Autodesk Inventor part; units mm, degrees
ref_plane "YZ Plane" through (0, 0, 0) normal (1, 0, 0) x (0, 1, 0)
ref_plane "XZ Plane" through (0, 0, 0) normal (0, 1, 0) x (-1, 0, 0)
ref_plane "XY Plane" through (0, 0, 0) normal (0, 0, 1) x (1, 0, 0)
sketch "Sketch1" plane through (0, 0, 0) normal (0, 1, 0) x (-1, 0, 0)
  circle A0 centre (0, -139.7) radius 3.3782
  line L0 (6.35, -37.5671) -> (6.35, -393.6488)
  line L1 (-6.35, -37.5671) -> (-6.35, -393.7)
  circle A1 centre (193.0245, -202.0047) radius 3.3782
  circle A2 centre (202.0047, -193.0245) radius 3.3782
  line L2 (269.2628, -287.2233) -> (16.4197, -34.3803)
  line L3 (287.2233, -269.2628) -> (34.3803, -16.4197)
  circle A3 centre (94.1906, -103.1708) radius 3.3782
  circle A4 centre (103.1708, -94.1906) radius 3.3782
  circle A5 centre (139.7, 0) radius 3.3782
  line L4 (133.35, 0) -> (133.35, 6.35)
  line L5 (273.05, 6.35) -> (273.05, 0)
  line L6 (37.5671, -6.35) -> (393.6488, -6.35)
  line L7 (37.5671, 6.35) -> (393.7, 6.35)
  line L8 (146.05, 0) -> (146.05, 6.35)
  circle A6 centre (277.5195, -270.2276) radius 3.3782
  circle A7 centre (270.2276, -277.5195) radius 3.3782
  arc A8 (269.2628, -287.2233) -> (287.2233, -269.2628) centre (0, 0) ccw
  circle A9 centre (0, -387.35) radius 3.3782
  arc A10 (0, -393.7) -> (6.35, -393.6488) centre (0, 0) ccw
  line L9 (-6.35, -393.7) -> (0, -393.7)
  circle A11 centre (0, -279.4) radius 3.3782
  arc A12 (6.35, -37.5671) -> (16.4197, -34.3803) centre (0, 0) ccw
  arc A13 (34.3803, -16.4197) -> (37.5671, -6.35) centre (0, 0) ccw
  circle A14 centre (0, 0) radius 14.2875
  line L10 (38.1, 0) -> (38.1, 12.8556) construction
  arc A15 (-6.214, 37.5898) -> (-37.5898, 6.214) centre (0, 0) ccw
  arc A16 (37.5671, 6.35) -> (-6.35, -37.5671) centre (0, 0) ccw
  circle A17 centre (387.35, 0) radius 3.3782
  line L11 (393.7, 0) -> (393.7, 6.35)
  circle A18 centre (279.4, 0) radius 3.3782
  line L12 (285.75, 6.35) -> (285.75, 0)
  arc A19 (393.6488, -6.35) -> (393.7, 0) centre (0, 0) ccw
  line L13 (0, -285.75) -> (-6.35, -285.75)
  line L14 (-6.35, -273.05) -> (0, -273.05)
  circle A20 centre (0, -336.55) radius 3.3782
  circle A21 centre (241.5985, -234.3065) radius 3.3782
  circle A22 centre (234.3065, -241.5985) radius 3.3782
  circle A23 centre (336.55, 0) radius 3.3782
  dimension "d2" = 12.7
  dimension "d3" = 12.7
  dimension "d4" = 38.1
  dimension "d6" = 38.1
  dimension "d7" = 6.35
  dimension "d8" = 6.35
  dimension "d9" = 6.35
  dimension "d10" = 12.7
  dimension "d11" = 12.7
  dimension "d12" = 95.25
  dimension "d13" = 6.7564
  dimension "d14" = 6.7564
  dimension "d15" = 6.7564
  dimension "d16" = 6.35
  dimension "d17" = 6.7564
  dimension "d18" = 6.35
  dimension "d19" = 6.35
  dimension "d20" = 6.7564
  dimension "d21" = 6.7564
  dimension "d22" = 6.7564
  dimension "d23" = 6.35
  dimension "d24" = 6.7564
  dimension "d25" = 28.575
  dimension "d28" = 38.1
  dimension "d30" = 6.35
  dimension "d31" = 139.7
  dimension "d34" = 6.35
  dimension "d37" = 277.5195
  dimension "d38" = 270.2276
  dimension "d39" = 7.2919
  dimension "d40" = 7.2919
  dimension "d41" = 393.7
  dimension "d42" = 393.7
  dimension "d43" = 6.35
  dimension "d44" = 12.7
  dimension "d45" = 6.7564
  dimension "d46" = 6.35
  dimension "d47" = 6.7564
  dimension "d48" = 6.7564
  dimension "d49" = 393.7
  dimension "d50" = 6.35
  dimension "d51" = 6.7564
  dimension "d52" = 6.35
  dimension "d54" = 6.7564
  dimension "d55" = 6.7564
  dimension "d56" = 6.7564
  dimension "d57" = 50.8
  dimension "d58" = 50.8
  dimension "d59" = 50.8
  dimension "d60" = 7.5438
  dimension "d61" = 7.5438
  dimension "d62" = 7.5438
  dimension "d63" = 7.5438
  dimension "d64" = 50.8
extrude "Extrusion1" add sketch "Sketch1" along normal blind 6.35
sketch "Sketch7" plane through (0, 6.35, 0) normal (0, 1, 0) x (1, 0, 0)
  circle A0 centre (0, 0) radius 9.5
  circle A1 centre (0, 0) radius 14.2875
  dimension "d99" = 19
extrude "Extrusion6" add sketch "Sketch7" against normal blind 6.35
sketch "Sketch9" plane through (0, 6.35, 0) normal (0, 1, 0) x (1, 0, 0)
  circle A0 centre (0, 139.7) radius 3.3782
  circle A1 centre (0, 279.4) radius 3.3782
  arc A2 (104.14, 347.9822) -> (104.1415, 56.1583) centre (110.49, 202.0703) ccw
  circle A3 centre (110.49, 202.0703) radius 146.05
  dimension "d102" = 0
  dimension "d103" = 0
  dimension "d104" = 0
extrude "Extrusion7" cut sketch "Sketch9" against normal blind 25.4
sketch "Sketch10" plane through (0, 6.35, 0) normal (0, 1, 0) x (1, 0, 0)
  arc A0 (6.35, 304.4688) -> (-6.35, 289.7003) centre (110.49, 202.0703) ccw
  line L0 (-6.35, 393.6488) -> (-6.35, 289.7003)
  arc A1 (-6.35, 114.4403) -> (6.35, 99.6717) centre (110.49, 202.0703) ccw
  line L1 (-6.35, 114.4403) -> (-6.35, 37.5671)
  arc A2 (-6.35, 37.5671) -> (-16.4197, 34.3803) centre (0, 0) ccw
  line L2 (-16.4197, 34.3803) -> (-269.2628, 287.2233)
  arc A3 (-269.2628, 287.2233) -> (-287.2233, 269.2628) centre (0, 0) ccw
  line L3 (-287.2233, 269.2628) -> (-34.3803, 16.4197)
  arc A4 (-34.3803, 16.4197) -> (-37.5671, 6.35) centre (0, 0) ccw
  line L4 (-37.5671, 6.35) -> (-393.6488, 6.35)
  arc A5 (-393.6488, 6.35) -> (-393.7, 0) centre (0, 0) ccw
  line L5 (-393.7, 0) -> (-393.7, -6.35)
  line L6 (-393.7, -6.35) -> (-37.5671, -6.35)
  arc A6 (-37.5671, -6.35) -> (6.35, 37.5671) centre (0, 0) ccw
  line L7 (6.35, 37.5671) -> (6.35, 99.6717)
  circle A7 centre (-270.2276, 277.5195) radius 3.3782
  circle A8 centre (-277.5195, 270.2276) radius 3.3782
  circle A9 centre (-234.3065, 241.5985) radius 3.3782
  circle A10 centre (-241.5985, 234.3065) radius 3.3782
  circle A11 centre (-387.35, 0) radius 3.3782
  circle A12 centre (-336.55, 0) radius 3.3782
  circle A13 centre (-139.7, 0) radius 3.3782
  circle A14 centre (-279.4, 0) radius 3.3782
  circle A15 centre (-94.1906, 103.1708) radius 3.3782
  circle A16 centre (-103.1708, 94.1906) radius 3.3782
  circle A17 centre (-193.0245, 202.0047) radius 3.3782
  circle A18 centre (-202.0047, 193.0245) radius 3.3782
  line L8 (-6.35, 114.4403) -> (-72.0725, 202.0703)
  line L9 (-6.35, 310.8669) -> (-129.1599, 147.1204)
  line L10 (-80.01, 191.4869) -> (-6.35, 93.2736)
  line L11 (-6.35, 289.7003) -> (-72.0725, 202.0703)
  line L12 (-80.01, 191.4869) -> (-120.0885, 138.049)
extrude "Extrusion8" add sketch "Sketch10" against normal blind 6.35 contours L0 L11 L8 L1 L10 L12 L2 L9
sketch "Sketch11" plane through (0, 6.35, 0) normal (0, 1, 0) x (1, 0, 0)
  circle A0 centre (-109.7506, 109.7506) radius 3.3782
  circle A1 centre (-133.5483, 133.5483) radius 3.3782
  circle A2 centre (-188.8658, 0) radius 3.3782
  circle A3 centre (-155.2108, 0) radius 3.3782
  circle A4 centre (-43.7228, 32.9465) radius 1.905
  circle A5 centre (-44.8017, 50.4305) radius 1.905
  line L0 (-26.4805, 78.1922) -> (-75.4609, 19.8196)
  line L1 (-59.4084, 6.35) -> (-75.4609, 19.8196)
  line L2 (-10.428, 64.7226) -> (-59.4084, 6.35)
  line L3 (-26.4805, 78.1922) -> (-10.428, 64.7226)
  circle A6 centre (-181.5311, 184.15) radius 1.7145
  circle A7 centre (-181.5311, 0) radius 1.7145
  line L4 (-189.0718, 209.55) -> (-173.9905, 209.55) construction
  line L5 (-189.0718, 209.55) -> (-189.0718, -6.35) construction
  line L6 (-173.9905, -6.35) -> (-189.0718, -6.35) construction
  line L7 (-173.9905, 209.55) -> (-173.9905, -6.35) construction
  circle A8 centre (-61.4602, 24.6503) radius 3.175
  circle A9 centre (-47.1743, 41.6757) radius 3.175
extrude "Extrusion9" cut sketch "Sketch11" against normal through all contours A0 | A1 | A2 | A3 | A4 | A5 | A6 | A7
equation "\"d60\" = d63"
equation "\"d61\" = d62"
properties part number "Bearing Mount Top" material "Aluminum 6061"
Work out the finished part from the listing and answer in its coordinate system (mm). A direction names the side the tool comes from. Round coordinates to 2 decimals unless told otherwise and drop trailing zeros. Order: outer loops, then holes, each group sorted by start corner. A loop starts at its lowest first (then second) coordinate and runs counter-clockwise, first axis right, second up.
Q1. Find the intervals of material crossed by line 1 along Z through (x, y) = (-97, 4.75); line 2 along X through (y, z) = (0.5, -163); line 3 along Z through (x, y) = (0, 4.5), in increasing order.
Solution:
line 1: z = -190 to -168.83, -114.96 to -105.05, -101.29 to -79.04, -6.35 to 6.35
line 2: x = -180.96 to -145.04, -117.25 to -101.38, -58.64 to -42.77
line 3: z = -393.7 to -390.73, -383.97 to -339.93, -333.17 to -297.58, -106.56 to -9.5, 9.5 to 38.1
Q2. Given pin 1 Ø1.9 at (y, z) = (1.5, -57.5) entering from +X; pin 2 Ø9 at (x, z) = (-277.52, -270.23) entering from +Y; pin 3 Ø1.5 at (x, y) = (-10, 3) entering from +Z; pin 4 Ø1 at (y, z) = (2, -282.5) entering from +X, each flat-ended and moving along its own axis, determine where each tip first touches the part or whether it passes through.
Solution:
pin 1: stops at x = 6.35
pin 2: stops at y = 6.35
pin 3: stops at z = 36.96
pin 4: stops at x = -11.38
Q3. A tool of negligible diameter and unlimited length cuts with its end or side. For faces 5 (the flat face through (-200.19, 3.13, -218.15)), 6 (the flat face through (-38.75, 3.22, -246.5)), 7 (the cylindrical face through (27.17, 3.13, 26.71)), 8 (the flat face through (-162.57, 3.13, -144.61)), 9 (the flat face through (-99.8, 3.2, -165.1)), from which of +Z, -Z, +X, -X, +Y, -Y can it reach the whole face along a straight path? Write none if from no direction.
Solution:
face 5: -Z, +Y, -Y
face 6: +X, +Y, -Y
face 7: +Z, +X, +Y, -Y
face 8: -X, +Y, -Y
face 9: +Y, -Y
Q4. A cutting plane is placed at B-B, the plane y = 3. Count the separate pieces of the cut face and the enclosed holes in it, then the cut area to 3 significant figures.
Solution:
separate pieces: 1
enclosed holes: 24
area: 23,200 mm2
Q5. A cutting plane is placed at A-A, the plane z = -213. Determine the outline of the cut face in (x, y).
Solution:
outline: (-230.96, 0) - (-195.04, 0) - (-195.04, 6.35) - (-230.96, 6.35) - close; (-79.75, 0) - (-63.88, 0) - (-63.88, 6.35) - (-79.75, 6.35) - close
Q6. The mould has two halves that part along Z. Classify faces 1 (the flat face through (-115, 6.35, -99)), 2 (the flat face through (-67, 3, -230)), 3 (the cylindrical face through (-0.16, 3.22, -297.4)), 4 (the flat face through (-38.75, 3.22, -157.64)): pulls with the +Z half, pulls with the -Z half, needs draft (parallel to the pull), parting line crosses it, or undercut.
Solution:
face 1: needs draft
face 2: pulls with the -Z half
face 3: undercut
face 4: undercut
